Geometry check sheet. Reference: the model listing, model coordinates, mm. Round coordinates to 2 decimals unless told otherwise and drop trailing zeros. Order: outer loops, then holes, each group sorted by start corner. A loop starts at its lowest first (then second) coordinate and runs counter-clockwise, first axis right, second up.
```python
from build123d import *

# Parameters (mm, degrees)
CROQUIS1_R                   = 4.5
CROQUIS1_R_2                 = 12
SALIENTE_EXTRUIR1_DEPTH      = 3
TALADRO_DE_MARGEN_PARA_M41_D = 4.5
TALADRO_DE_MARGEN_PARA_M42_D = 4.5
TALADRO_DE_MARGEN_PARA_M32_D = 3.4


with BuildPart() as part:
    # Croquis1 → Saliente-Extruir1 (new, symmetric)
    with BuildSketch(Plane(origin=(0, 0, 0), x_dir=(1, 0, 0), z_dir=(0, 1, 0))):
        Polygon((-54, -109), (-25, -109), (-25, -115), (25, -115), (25, -109), (54, -109), (54, -30), (60, -30), (60, 30), (54, 30), (54, 109), (25, 109), (25, 115), (-25, 115), (-25, 109), (-54, 109), (-54, 30), (-60, 30), (-60, -30), (-54, -30), align=None)
        with Locations(Location((0, -65, 0), (0, 0, 270))):
            Circle(CROQUIS1_R, mode=Mode.SUBTRACT)
        with Locations(Location((0, 80, 0), (0, 0, 270))):
            Circle(CROQUIS1_R_2, mode=Mode.SUBTRACT)
    extrude(amount=SALIENTE_EXTRUIR1_DEPTH, both=True)

    # Taladro de margen para M41 (through all)
    with Locations(Plane(origin=(0, 3, 0), x_dir=(1, 0, 0), z_dir=(0, 1, 0))):
        with Locations((-12.5, -77.5), (-12.5, -52.5), (12.5, -52.5), (12.5, -77.5)):
            Hole(TALADRO_DE_MARGEN_PARA_M41_D / 2)

    # Taladro de margen para M42 (through all)
    with Locations(Plane(origin=(0, 3, 0), x_dir=(1, 0, 0), z_dir=(0, 1, 0))):
        with Locations((-40, 80), (-40, -65), (40, -65), (40, 80)):
            Hole(TALADRO_DE_MARGEN_PARA_M42_D / 2)

    # Taladro de margen para M32 (through all)
    with Locations(Plane(origin=(0, -3, 0), x_dir=(-1, 0, 0), z_dir=(0, -1, 0))):
        with Locations((-15.5, 64.5), (-15.5, 95.5), (15.5, 95.5), (15.5, 64.5)):
            Hole(TALADRO_DE_MARGEN_PARA_M32_D / 2)


solid = part.part
```
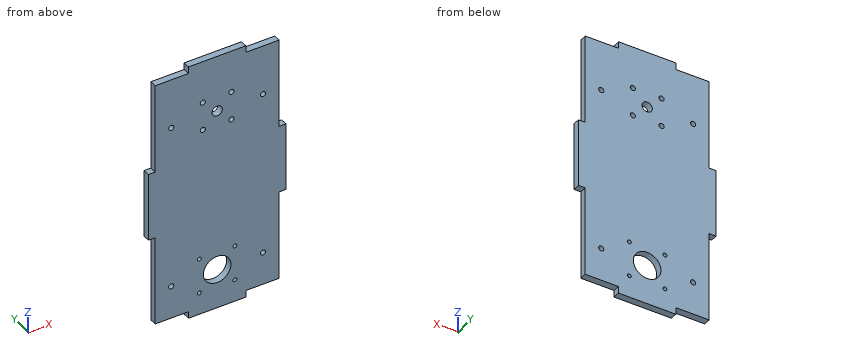
(1) Sectioned sample at A-A, the plane z = -80. Record the cut outline in (x, y).
Returned:
outline: (-54, -3) - (-42.25, -3) - (-42.25, 3) - (-54, 3) - close; (-37.75, -3) - (-12, -3) - (-12, 3) - (-37.75, 3) - close; (12, -3) - (37.75, -3) - (37.75, 3) - (12, 3) - close; (42.25, -3) - (54, -3) - (54, 3) - (42.25, 3) - close
(2) Sectioned sample at B-B, the plane y = -0.95. Give the number of separate pieces and of enclosed holes in the cut face, and give its area (3 significant figures).
Returned:
separate pieces: 1
enclosed holes: 14
area: 24,200 mm2
(3) Depth check by flat-ended pin: P1, Ø2, axis at y = 1, z = -63, coming from the -X side; P2, Ø3, axis at x = 42, y = 0, coming from the +Z side; P3, Ø1.8, axis at y = 1, z = 111.5, coming from the -X side. Enter the tip coordinate at first touch or a pass-through.
Returned:
P1: stops at x = -54
P2: stops at z = 109
P3: stops at x = -25
(4) Sectioned sample at C-C, the plane x = -40. Record the cut outline in (y, z), and give its area (3 significant figures).
Returned:
outline: (-3, -109) - (3, -109) - (3, -82.25) - (-3, -82.25) - close; (-3, -77.75) - (3, -77.75) - (3, 62.75) - (-3, 62.75) - close; (-3, 67.25) - (3, 67.25) - (3, 109) - (-3, 109) - close
area: 1,250 mm2
(5) Material ranges on line 1 (Z direction, x = 40, y = -0.05); line 2 (X direction, y = -0.4, z = 52.5); line 3 (X direction, y = 0.3, z = -64.5), recorded low to high.
Returned:
line 1: z = -109 to -82.25, -77.75 to 62.75, 67.25 to 109
line 2: x = -54 to -14.75, -10.25 to 10.25, 14.75 to 54
line 3: x = -54 to -17.2, -13.8 to 13.8, 17.2 to 54
(6) Sectioned sample at D-D, the plane z = 65. Record the cut outline in (x, y).
Returned:
outline: (-54, -3) - (-42.25, -3) - (-42.25, 3) - (-54, 3) - close; (-37.75, -3) - (-4.5, -3) - (-4.5, 3) - (-37.75, 3) - close; (4.5, -3) - (37.75, -3) - (37.75, 3) - (4.5, 3) - close; (42.25, -3) - (54, -3) - (54, 3) - (42.25, 3) - close
